Check sheet for the modelled part. Datum: model origin and axes. Units: mm. A direction names the side the tool comes from. Coordinates: 2 decimals unless noted, no trailing zeros. Loops run counter-clockwise (first coordinate to the right, second up) from the corner with the lowest first, then second, coordinate; pieces in that order, holes last.
```python
from build123d import *

# Parameters (mm, degrees)
ESQUISSE1_W                  = 94
ESQUISSE1_H                  = 64
BOSS_EXTRU_1_DEPTH           = 3
ESQUISSE2_R                  = 26
BOSS_EXTRU_2_DEPTH           = 7
BOSS_EXTRU_3_DEPTH           = 22.5
BOSS_EXTRU_3_DEPTH_BACK      = 22.5
ENL_V_MAT_EXTRU_1_DEPTH      = 173.665138346
ENL_V_MAT_EXTRU_1_DEPTH_BACK = 173.665138346
ESQUISSE4_W                  = 86
ESQUISSE4_H                  = 39
ENL_V_MAT_EXTRU_2_DEPTH      = 143.697231928
ENL_V_MAT_EXTRU_2_DEPTH_BACK = 143.697231928
ESQUISSE5_R                  = 4
ENL_V_MAT_EXTRU_3_DEPTH      = 3
CHANFREIN1_SIZE              = 6


with BuildPart() as part:
    # Esquisse1 → Boss.-Extru.1 (new body)
    with BuildSketch(Plane.XY):
        with Locations((47, 32)):
            Rectangle(ESQUISSE1_W, ESQUISSE1_H)
    extrude(amount=BOSS_EXTRU_1_DEPTH)

    # Esquisse2 → Boss.-Extru.2 (add)
    with BuildSketch(Plane.XY.offset(3)):
        with Locations((47, 32)):
            Circle(ESQUISSE2_R)
    extrude(amount=BOSS_EXTRU_2_DEPTH)

    # Esquisse3 → Boss.-Extru.3 (add, two sides: drawn at the far end of the back side and taken through both)
    with BuildSketch(Plane(origin=(0, 32, 0), x_dir=(1, 0, 0), z_dir=(0, 1, 0)).offset(-BOSS_EXTRU_3_DEPTH_BACK)):
        with BuildLine():
            Line((73, -10), (73, -19))
            Line((73, -19), (65, -25))
            Line((65, -25), (25, -80))
            ThreePointArc((25, -80), (12.5, -92.5), (0, -80))
            Line((0, -80), (0, -40))
            Line((0, -40), (-29, -30))
            ThreePointArc((-29, -30), (-37, -22), (-29, -14))
            Line((-29, -14), (21, -10))
            Line((21, -10), (73, -10))
        make_face()
    extrude(amount=BOSS_EXTRU_3_DEPTH + BOSS_EXTRU_3_DEPTH_BACK)

    # Esquisse4 → Enlèv. mat.-Extru.1 (cut, two sides: drawn at the far end of the back side and taken through both)
    with BuildSketch(Plane(origin=(94, 0, 0), x_dir=(0, 0, -1), z_dir=(1, 0, 0)).offset(-ENL_V_MAT_EXTRU_1_DEPTH_BACK)):
        with Locations((-56, 32)):
            Rectangle(ESQUISSE4_W, ESQUISSE4_H)
    extrude(amount=ENL_V_MAT_EXTRU_1_DEPTH + ENL_V_MAT_EXTRU_1_DEPTH_BACK, mode=Mode.SUBTRACT)

    # Esquisse5 → Enlèv. mat.-Extru.2 (cut, two sides: drawn at the far end of the back side and taken through both)
    with BuildSketch(Plane.XZ.offset(-9.5).offset(-ENL_V_MAT_EXTRU_2_DEPTH_BACK)):
        with Locations(Location((12.5, 80, 0), (0, 0, 270))):
            Circle(ESQUISSE5_R)
    extrude(amount=ENL_V_MAT_EXTRU_2_DEPTH + ENL_V_MAT_EXTRU_2_DEPTH_BACK, mode=Mode.SUBTRACT)

    # Esquisse6 → Enlèv. mat.-Extru.3 (cut)
    with BuildSketch(Plane(origin=(0, 0, 0), x_dir=(-1, 0, 0), z_dir=(0, 0, -1))):
        with BuildLine():
            Line((-86.5, 59), (-81.5, 59))
            ThreePointArc((-81.5, 59), (-77, 54.5), (-81.5, 50))
            Line((-81.5, 50), (-86.5, 50))
            ThreePointArc((-86.5, 50), (-91, 54.5), (-86.5, 59))
        make_face()
        with BuildLine():
            Line((-7.5, 59), (-12.5, 59))
            ThreePointArc((-12.5, 59), (-17, 54.5), (-12.5, 50))
            Line((-12.5, 50), (-7.5, 50))
            ThreePointArc((-7.5, 50), (-3, 54.5), (-7.5, 59))
        make_face()
        with BuildLine():
            Line((-7.5, 5), (-12.5, 5))
            ThreePointArc((-12.5, 5), (-17, 9.5), (-12.5, 14))
            Line((-12.5, 14), (-7.5, 14))
            ThreePointArc((-7.5, 14), (-3, 9.5), (-7.5, 5))
        make_face()
        with BuildLine():
            Line((-86.5, 5), (-81.5, 5))
            ThreePointArc((-81.5, 5), (-77, 9.5), (-81.5, 14))
            Line((-81.5, 14), (-86.5, 14))
            ThreePointArc((-86.5, 14), (-91, 9.5), (-86.5, 5))
        make_face()
    extrude(amount=-ENL_V_MAT_EXTRU_3_DEPTH, mode=Mode.SUBTRACT)

    # Chanfrein1
    chanfrein1_edges = [part.edges().sort_by_distance(p)[0] for p in [
        (0, 64, 1.5),
        (94, 64, 1.5),
        (94, 0, 1.5),
        (0, 0, 1.5),
    ]]
    chamfer(chanfrein1_edges, length=CHANFREIN1_SIZE)


solid = part.part
```
1) Section check A-A on z = 22. Enter the section's corners in (x, y), plus the area to 3 significant figures.
Answer sheet:
outline: (-37, 9.5) - (69, 9.5) - (69, 12.5) - (-37, 12.5) - close; (-37, 51.5) - (69, 51.5) - (69, 54.5) - (-37, 54.5) - close
area: 636 mm2
2) Set-up check for faces 4 (the cylindrical face through (3, 54.4, 1.5)), 5 (the flat face through (19, 9.5, 42)), 6 (the flat face through (0, 53, 60)), 7 (the flat face through (73, 32, 12)), 8 (the flat face through (10, 5, 1)): record each of +Z, -Z, +X, -X, +Y, -Y from which the full face is reachable in a straight line by a thin tool's end or side.
Answer sheet:
face 4: -Z
face 5: +Z, +X, -X, -Y
face 6: +Z, -X, +Y, -Y
face 7: +Z, +X, +Y, -Y
face 8: +Z, -Z
3) Section check B-B on y = 11. Enter the section's corners in (x, z), plus the area to 3 significant figures.
Answer sheet:
outline: (-29, 14) - (21, 10) - (31.67, 10) - (31.67, 3) - (16.74, 3) - (16.74, 0) - (77.26, 0) - (77.26, 3) - (62.33, 3) - (62.33, 10) - (73, 10) - (73, 19) - (65, 25) - (25, 80) arc R12.5 ccw to (0, 80) - (0, 40) - (-29, 30) arc R8 ccw to start; (0, 0) - (3.26, 0) - (3.26, 3) - (0, 3) - close; (90.74, 0) - (94, 0) - (94, 3) - (90.74, 3) - close; hole circle Ø8 at (12.5, 80)
area: 4,880 mm2
4) Mould release check, pull along Y, two halves, no side actions. Record for faces 1 (the flat face through (19, 54.5, 42)), 2 (the flat face through (25, 47, 3)), 3 (the flat face through (84, 50, 1)): +Y half, -Y half, draft (parallel to the pull), parting line (faces both ways), or undercut.
Answer sheet:
face 1: +Y half
face 2: draft
face 3: undercut
5) Depth check by flat-ended pin: pin 1 (2 mm diameter, centred on x = 30, z = 65.5, fed in from -Y); pin 2 (10 mm diameter, centred on y = 17, z = 68.5, fed in from -X); pin 3 (4 mm diameter, centred on y = 52.5, z = 36.5, fed in from +X). Enter the tip coordinate at first touch or a pass-through.
Answer sheet:
pin 1: stops at y = 9.5
pin 2: stops at x = 0
pin 3: stops at x = 58.09
6) Scan lines: line 1 (X direction, y = 52.75, z = 80); line 2 (Y direction, x = 25, z = 38.5); line 3 (Z direction, x = 52, y = 26). Record each from-to range of solid material in increasing order.
Answer sheet:
line 1: x = 0 to 8.5, 16.5 to 25
line 2: y = 9.5 to 12.5, 51.5 to 54.5
line 3: z = 0 to 13
7) Section check C-C on x = 37. Enter the section's corners in (y, z), plus the area to 3 significant figures.
Answer sheet:
outline: (0, 0) - (64, 0) - (64, 3) - (56, 3) - (56, 10) - (54.5, 10) - (54.5, 63.5) - (51.5, 63.5) - (51.5, 13) - (12.5, 13) - (12.5, 63.5) - (9.5, 63.5) - (9.5, 10) - (8, 10) - (8, 3) - (0, 3) - close
area: 966 mm2
8) Section check D-D on x = 14.5. Enter the section's corners in (y, z).
Answer sheet:
outline: (0, 0) - (5.47, 0) - (5.47, 3) - (0, 3) - close; (9.5, 10.52) - (54.5, 10.52) - (54.5, 76.54) - (51.5, 76.54) - (51.5, 13) - (12.5, 13) - (12.5, 76.54) - (9.5, 76.54) - close; (9.5, 83.46) - (12.5, 83.46) - (12.5, 92.34) - (9.5, 92.34) - close; (13.53, 0) - (50.47, 0) - (50.47, 3) - (13.53, 3) - close; (51.5, 83.46) - (54.5, 83.46) - (54.5, 92.34) - (51.5, 92.34) - close; (58.53, 0) - (64, 0) - (64, 3) - (58.53, 3) - close
